CAD build for the part. Positions are in the model's coordinates, mm. A direction names the side the tool comes from. Coordinates: 2 decimals unless noted, no trailing zeros. Order: outer loops, then holes, each group sorted by start corner. A loop starts at its lowest first (then second) coordinate and runs counter-clockwise, first axis right, second up. Notation, with made-up numbers: (32.25, -37.75) - (54.25, -37.75) arc R8 cw to (54.25, -28.75) - close; hole circle Ø9 at (-30.5, -25.75). An arc over 180 degrees is marked (long way). Return JSON: item names as keys, results as strings.
Autodesk Fusion 360 part; units mm, degrees
sketch "Sketch3" plane through (0, 0, 0) normal (0, 0, 1) x (-1, 0, 0)
  circle A0 centre (13, -13) radius 1
  circle A1 centre (13, 13) radius 1
  circle A2 centre (-13, 13) radius 1
  circle A3 centre (-13, -13) radius 1
  circle A4 centre (13, -13) radius 1.6
  circle A5 centre (13, 13) radius 1.6
  circle A6 centre (-13, 13) radius 1.6
  circle A7 centre (-13, -13) radius 1.6
  line L0 (17.5, -14.8) -> (17.5, 14.8)
  line L1 (17.5, 14.8) -> (15.3, 17)
  line L2 (15.3, 17) -> (-15.3, 17)
  line L3 (-15.3, 17) -> (-17.5, 14.8)
  line L4 (-17.5, 14.8) -> (-17.5, -14.8)
  line L5 (-17.5, -14.8) -> (-15.3, -17)
  line L6 (-15.3, -17) -> (15.3, -17)
  line L7 (15.3, -17) -> (17.5, -14.8)
  circle A8 centre (0, 0) radius 11.65
  circle A9 centre (0, 0) radius 8.65
  line L8 (8.5, 17) -> (-8.5, 17)
  line L9 (-8.5, 17) -> (-8.5, 12)
  line L10 (-8.5, 12) -> (8.5, 12)
  line L11 (8.5, 12) -> (8.5, 17)
  line L12 (8.5, -17) -> (-8.5, -17)
  line L13 (-8.5, -17) -> (-8.5, -12)
  line L14 (-8.5, -12) -> (8.5, -12)
  line L15 (8.5, -12) -> (8.5, -17)
  point P0 (17.5, -14.8)
  point P1 (15.3, -17)
  point P2 (17.5, 14.8)
  point P3 (15.3, 17)
  point P4 (-15.3, 17)
  point P5 (-17.5, 14.8)
  point P6 (-17.5, -14.8)
  point P7 (-15.3, -17)
  point P8 (-17.5, -8.8262)
  point P9 (-17.5, 8.8262)
  point P10 (-9, 17)
  point P11 (9, 17)
  point P12 (9, -17)
  point P13 (-9, -17)
  dimension "d26" = 3.2
  dimension "d27" = 3.2
  dimension "d28" = 3.2
  dimension "d29" = 3.2
  dimension "d30" = 23.3
  dimension "d31" = -3
  dimension "d38" = 5
  dimension "d39" = 0.5
  dimension "d40" = 0.5
  dimension "d41" = 0.5
  dimension "d42" = 5
  dimension "d43" = 0.5
extrude "Extrude6" add sketch "Sketch3" against normal blind 3 contours L6 L12 L13 L14 L15 | L2 L8 L9 L10 L11 makes body 1 at (2.8333, -15.3333, 0) makes body 2 at (-2.8333, 13.6667, 0)
extrude "Extrude3" add sketch "Sketch3" along normal blind 3 contours L0 L1 L2 L3 L4 L5 L6 L7 L9 L10 L11 L13 L14 L15 | L6 L12 L13 L14 L15 | L2 L8 L9 L10 L11 | A8 bodies 1 2
extrude "Extrude4" cut sketch "Sketch3" along normal blind 40 contours A8 bodies 1
extrude "Extrude5" add sketch "Sketch3" along normal blind 50 contours A8 bodies 1
sketch "Sketch4" plane through (17.5, 0, 0) normal (1, 0, 0) x (0, 1, 0)
  line L0 (-14.8, 0) -> (14.8, 0)
  line L1 (14.8, 0) -> (14.8, 3)
  line L2 (14.8, 3) -> (-14.8, 3)
  line L3 (-14.8, 3) -> (-14.8, 0)
  line L4 (1.289, 2.5498) -> (9.3, 0)
  line L5 (-1.289, 2.5498) -> (-9.3, 0)
  arc A0 (1.289, 2.5498) -> (-1.289, 2.5498) centre (0, -1.5) ccw
  line L6 (0, 0) -> (0, -1.5) construction
  dimension "d50" = 4.25
  dimension "d51" = 5.5
  dimension "d52" = 5.5
  dimension "d54" = 1.5
extrude "Extrude7" cut sketch "Sketch4" along normal through all contours L0 L4 L5 A0 bodies 1
Item 1: Band-saw the part on D-D, the plane x = -1. List the corners of the cut face in (y, z), then the cut area to 3 significant figures.
Findings below:
{"outline": "(-17, -3) - (-12, -3) - (-12, 0) - (-8.59, 0) - (-8.59, 50) - (-11.61, 50) - (-11.61, 3) - (-17, 3) - close; (8.59, 0) - (12, 0) - (12, -3) - (17, -3) - (17, 3) - (11.61, 3) - (11.61, 50) - (8.59, 50) - close", "area": "364 mm²"}
Item 2: Band-saw the part on C-C, the plane y = 13. List the corners of the cut face in (x, z), then the cut area to 3 significant figures.
Findings below:
{"outline": "(-17.5, 0) - (-14.6, 0) - (-14.6, 3) - (-17.5, 3) - close; (-11.4, 0) - (-8.5, 0) - (-8.5, -3) - (8.5, -3) - (8.5, 0) - (11.4, 0) - (11.4, 3) - (-11.4, 3) - close; (14.6, 0) - (17.5, 0) - (17.5, 3) - (14.6, 3) - close", "area": "137 mm²"}
Item 3: Band-saw the part on A-A, the plane y = 0. List the corners of the cut face in (x, z).
Findings below:
{"outline": "(-17.5, 0) - (-8.65, 0) - (-8.65, 50) - (-11.65, 50) - (-11.65, 3) - (-17.5, 3) - close; (8.65, 0) - (17.5, 0) - (17.5, 3) - (11.65, 3) - (11.65, 50) - (8.65, 50) - close"}
Item 4: Band-saw the part on B-B, the plane x = -13. List the corners of the cut face in (y, z).
Findings below:
{"outline": "(-17, 0) - (-14.6, 0) - (-14.6, 3) - (-17, 3) - close; (-11.4, 0) - (11.4, 0) - (11.4, 3) - (-11.4, 3) - close; (14.6, 0) - (17, 0) - (17, 3) - (14.6, 3) - close"}
Item 5: Which spindle directions (+Z, -Z, +X, -X, +Y, -Y) get a long thin tool onto all of the face, cutting with end or side? Do faces 4 (the flat face through (0, -12, -1)), 5 (the flat face through (8.5, 15, -1)), 6 (the flat face through (12, 0, 3)). Say none if no direction does.
Findings below:
{"face 4": "-Z, +X, -X", "face 5": "-Z, +X, +Y, -Y", "face 6": "+Z"}
Item 6: Wall check: L1, parallel to X at y = 13, z = 1; L2, parallel to Y at x = -13, z = 1.6; L3, parallel to Y at x = 0, z = 33. Give the ranges that are in metal, low to high. Write a range as [from, to].
Findings below:
{"L1": "x = [-17.5, -14.6], [-11.4, 11.4], [14.6, 17.5]", "L2": "y = [-17, -14.6], [-11.4, 11.4], [14.6, 17]", "L3": "y = [-11.65, -8.65], [8.65, 11.65]"}
Item 7: Drop flat-ended pins along their axis: P1, Ø4, axis at x = -4.5, z = 40.5, coming from the -Y side; P2, Ø8, axis at y = 10.5, z = 27, coming from the +X side; P3, Ø5, axis at x = 13, y = 13, coming from the +Z side; P4, Ø1, axis at x = 7, y = -4, coming from the -Z side. Give the stop position or say it passes through.
Findings below:
{"P1": "stops at y = -11.38", "P2": "stops at x = 9.67", "P3": "stops at z = 3", "P4": "passes through"}
Item 8: Mould opens along X. For faces 1 (the cylindrical face through (-11.4, 13.07, 1.48)), 2 (the flat face through (-8.5, -14, -1)), 3 (the flat face through (8.5, -15, -1)) say: released by +X, released by -X, zero draft, split by the parting line, or undercut.
Findings below:
{"face 1": "undercut", "face 2": "released by -X", "face 3": "released by +X"}
